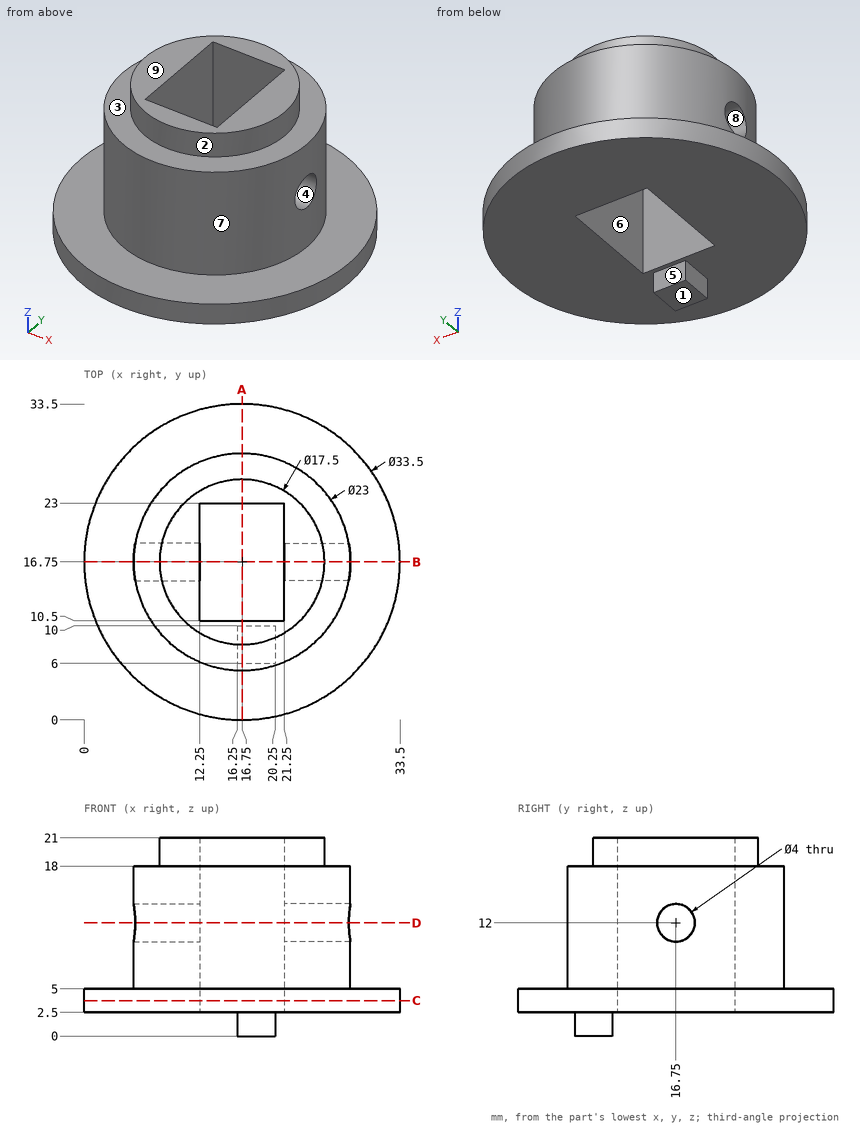
The figure shows three views and two pictorial views of one solid part (mm, origin at its lowest corner). Answer the questions. A direction names the side the tool comes from. Coordinates: 2 decimals unless noted, no trailing zeros. Loops run counter-clockwise (first coordinate to the right, second up) from the corner with the lowest first, then second, coordinate; pieces in that order, holes last. Notation, with made-up numbers: (73.5, -39) - (116.5, -39) arc R17 ccw to (116.5, -16) - close; hole circle Ø6 at (44, -35.5). An arc over 180 degrees is marked (long way). Use a Markdown table: item, result. Add a question column.
1) Find the intervals of material crossed by line 1 (Z direction, x = 10.25, y = 16.75); line 2 (Z direction, x = 3, y = 15); line 3 (Y direction, x = 24.75, z = 12), in increasing order.
2) For the marked faces 5, 6, 7, 8 and 9, determine the directions among +Z, -Z, +X, -X, +Y, -Y from which every point of the face is accessible in a straight line to the end or side of a thin tool.
3) The mould has two halves that part along Z. Classify the marked faces 1, 2, 3 and 4: released by +Z, released by -Z, zero draft, split by the parting line, or undercut.
4) Given pin 1 (1.5 mm diameter, centred on x = 19.5, z = 7, fed in from -Y); pin 2 (12 mm diameter, centred on x = 7.5, y = 23, fed in from -Z); pin 3 (3 mm diameter, centred on y = 19, z = 16.5, fed in from +X); pin 4 (7 mm diameter, centred on x = 17.5, y = 21, fed in from +Z), each flat-ended and moving along its own axis, determine where each tip first touches the part or whether it passes through.
5) The part is cut by section A-A, the plane x = 16.75. Give the vertices of the cut face in (y, z).
6) The part is cut by section D-D, the plane z = 12. Give the vertices of the cut face in (x, y), and give its area (3 significant figures).
7) The part is cut by section B-B, the plane y = 16.75. Give the vertices of the cut face in (x, z), and give its area (3 significant figures).
8) The part is cut by section C-C, the plane z = 3.75. Give the vertices of the cut face in (x, y).
Here are the results:
| question | item | result |
|---|---|---|
| 1 | line 1 | z = 2.5 to 10, 14 to 21 |
| 1 | line 2 | z = 2.5 to 5 |
| 1 | line 3 | y = 8.49 to 14.75, 18.75 to 25.01 |
| 2 | face 5 | -Z, +X, -X, +Y |
| 2 | face 6 | +Z, -Z |
| 2 | face 7 | +Z |
| 2 | face 8 | +X, -X |
| 2 | face 9 | +Z, +X, -X, +Y, -Y |
| 3 | face 1 | released by -Z |
| 3 | face 2 | zero draft |
| 3 | face 3 | released by +Z |
| 3 | face 4 | undercut |
| 4 | pin 1 | stops at y = 5.43 |
| 4 | pin 2 | stops at z = 2.5 |
| 4 | pin 3 | stops at x = 28.23 |
| 4 | pin 4 | stops at z = 21 |
| 5 | outline | (0, 2.5) - (6, 2.5) - (6, 0) - (10, 0) - (10, 2.5) - (10.5, 2.5) - (10.5, 21) - (8, 21) - (8, 18) - (5.25, 18) - (5.25, 5) - (0, 5) - close; (23, 2.5) - (33.5, 2.5) - (33.5, 5) - (28.25, 5) - (28.25, 18) - (25.5, 18) - (25.5, 21) - (23, 21) - close |
| 6 | outline | (5.43, 14.75) arc R11.5 ccw to (28.07, 14.75) - (21.25, 14.75) - (21.25, 10.5) - (12.25, 10.5) - (12.25, 14.75) - close; (5.43, 18.75) - (12.25, 18.75) - (12.25, 23) - (21.25, 23) - (21.25, 18.75) - (28.07, 18.75) arc R11.5 ccw to start |
| 6 | area | 247 mm^2 |
| 7 | outline | (0, 2.5) - (12.25, 2.5) - (12.25, 10) - (5.25, 10) - (5.25, 5) - (0, 5) - close; (5.25, 14) - (12.25, 14) - (12.25, 21) - (8, 21) - (8, 18) - (5.25, 18) - close; (21.25, 2.5) - (33.5, 2.5) - (33.5, 5) - (28.25, 5) - (28.25, 10) - (21.25, 10) - close; (21.25, 14) - (28.25, 14) - (28.25, 18) - (25.5, 18) - (25.5, 21) - (21.25, 21) - close |
| 7 | area | 213 mm^2 |
| 8 | outline | circle Ø33.5 at (16.75, 16.75); hole (12.25, 10.5) - (21.25, 10.5) - (21.25, 23) - (12.25, 23) - close |
